For this review, take the finished solid that the model builds, in its own axes (mm). A direction names the side the tool comes from. Coordinates: 2 decimals unless noted, no trailing zeros. Loops run counter-clockwise (first coordinate to the right, second up) from the corner with the lowest first, then second, coordinate; pieces in that order, holes last. Notation, with made-up numbers: (-22.5, 74) - (10.5, 74) arc R34 ccw to (10.5, 113) - close; hole circle Ø7 at (17, 10). An arc over 180 degrees is marked (long way). Answer as a JSON object with one key per item and string values. Group by question number.
Item 1: We need section A-A (z = -3.75). Give the boundary of the cut face in (x, y), then the cut area to 3 significant figures.
Item 2: We need section B-B (z = -6). Give the boundary of the cut face in (x, y).
Item 3: Tool access review of faces 1 (the cylindrical face through (4.967, -1.564, -6.082)), 2 (the flat face through (2.6, 4.7, -5.08)), 3 (the flat face through (2.6, -4.7, -5.08)), 4 (the flat face through (-2.6, -4.7, -5.08)): name each direction out of +Z, -Z, +X, -X, +Y, -Y from which nothing blocks a thin tool from reaching the whole face with its end or side.
Item 4: To check wall thickness, follow line 1 (Y direction, x = 0, z = -5.8); line 2 (Y direction, x = 0, z = -2.3); line 3 (X direction, y = 2.75, z = -4). State the ranges of each line that lie inside material, in increasing order.
Item 5: Clearance check with flat-ended pins moving along their axes: pin 1 (1.1 mm diameter, centred on x = -2.5, y = 4.5, fed in from -Z); pin 2 (4 mm diameter, centred on y = 3.5, z = -4.5, fed in from +X); pin 3 (1.5 mm diameter, centred on y = -3, z = -1, fed in from -X). State where each tip first meets the part, or that it passes through.
from build123d import *

# Parameters (mm, degrees)
SKETCH1_R      = 3.1115
EXTRUDE1_DEPTH = 5.08
SKETCH2_R      = 5.207
SKETCH2_R_2    = 3.1115
EXTRUDE2_DEPTH = 2.54
FILLET1_R      = 0.508


with BuildPart() as part:
    # Sketch1 → Extrude1 (new body)
    with BuildSketch(Plane.XY):
        Polygon((3.182239214, 5.588), (-3.182239214, 5.588), (-6.408472518, 0), (-3.182239214, -5.588), (3.182239214, -5.588), (6.408472518, 0), align=None)
        Circle(SKETCH1_R, mode=Mode.SUBTRACT)
    extrude(amount=-EXTRUDE1_DEPTH)

    # Sketch2 → Extrude2 (add)
    with BuildSketch(Plane(origin=(0, 0, -5.08), x_dir=(-1, 0, 0), z_dir=(0, 0, -1))):
        with Locations(Location((0, 0, 0), (0, 0, 180))):
            Circle(SKETCH2_R)
        with Locations(Location((0, 0, 0), (0, 0, 180))):
            Circle(SKETCH2_R_2, mode=Mode.SUBTRACT)
    extrude(amount=EXTRUDE2_DEPTH)

    # Fillet1
    fillet1_edges = [part.edges().sort_by_distance(p)[0] for p in [
        (-4.795355866, 2.794, -5.08),
        (6.408472518, 0, -2.54),
        (3.182239214, -5.588, -2.54),
        (-3.182239214, -5.588, -2.54),
        (-6.408472518, 0, -2.54),
        (-3.182239214, 5.588, -2.54),
        (3.182239214, 5.588, -2.54),
        (-4.795355866, -2.794, -5.08),
        (0, -5.588, -5.08),
        (4.795355866, -2.794, -5.08),
        (-5.207, 0, -7.62),
        (4.795355866, 2.794, -5.08),
        (4.795355866, -2.794, 0),
        (0, -5.588, 0),
        (-4.795355866, -2.794, 0),
        (0, 5.588, -5.08),
        (-4.795355866, 2.794, 0),
        (0, 5.588, 0),
        (4.795355866, 2.794, 0),
    ]]
    fillet(fillet1_edges, radius=FILLET1_R)


solid = part.part
Check sheet entries:
{
 "1": {"outline": "(-6.26, -0.25) - (-3.33, -5.33) arc R0.51 ccw to (-2.89, -5.59) - (2.89, -5.59) arc R0.51 ccw to (3.33, -5.33) - (6.26, -0.25) arc R0.51 ccw to (6.26, 0.25) - (3.33, 5.33) arc R0.51 ccw to (2.89, 5.59) - (-2.89, 5.59) arc R0.51 ccw to (-3.33, 5.33) - (-6.26, 0.25) arc R0.51 ccw to start; hole circle Ø6.22 at (0, 0)", "area": "76.7 mm2"},
 "2": {"outline": "circle Ø10.41 at (0, 0); hole circle Ø6.22 at (0, 0)"},
 "3": {"face 1": "-Z", "face 2": "-Z, +X, +Y", "face 3": "-Z, +X, -Y", "face 4": "-Z, -X, -Y"},
 "4": {"line 1": "y = -5.21 to -3.11, 3.11 to 5.21", "line 2": "y = -5.59 to -3.11, 3.11 to 5.59", "line 3": "x = -4.82 to -1.46, 1.46 to 4.82"},
 "5": {"pin 1": "stops at z = -7.62", "pin 2": "stops at x = 5.54", "pin 3": "stops at x = -5.11"}
}
